Input: part model. Units: mm. Frame: model coordinates. A direction names the side the tool comes from. Round coordinates to 2 decimals unless told otherwise and drop trailing zeros. Loops run counter-clockwise (first coordinate to the right, second up) from the corner with the lowest first, then second, coordinate; pieces in that order, holes last. Notation, with made-up numbers: (-32, 20) -> (-15, 20) arc R16 ccw to (-15, 50) -> close; hole circle Ø6 at (25.25, 24). An arc over 180 degrees is marked (long way). Answer in a Markdown table with one row per item. Add a question column.
Q1. Reachability of faces 1 (the face through (10, 53.34, 10)), 2 (the face through (-22.33, 59.6, 21.93)), 3 (the face through (0.251, 9.396, 29.936)) from +Z, -Z, +X, -X, +Y, -Y: full face, straight path, thin tool, end or side. Return the list, or none.
Q2. Pin query (flat end, axial travel): pin 1 (4 mm diameter, centred on y = 5, z = -5.5, fed in from +X); pin 2 (6 mm diameter, centred on x = -3.5, y = 28, fed in from +Z); pin 3 (4 mm diameter, centred on x = -5.5, y = 2.5, fed in from +Z); pin 4 (8 mm diameter, centred on x = 0, z = -35.92, fed in from +Y). Return the tip coordinate at first contact, or that it passes through.
Q3. Mould query, pull axis X, two halves, no side actions, for faces 4 (the face through (-0.251, 9.396, -29.936)), 5 (the face through (-48.62, 59.6, -0.23)), 6 (the face through (13.52, 5.01, -18.16)). Classes: pulls with the +X half, pulls with the -X half, needs draft (parallel to the pull), parting line crosses it, or undercut.
Q4. Section C-C, the plane y = 38. Output: boundary loops of the cut face in (x, z) (3 decimals), and give its area (3 significant figures).
Q5. Ray query, L1, parallel to Y at x = -11, z = -9.5; L2, parallel to Z at x = 0, y = 26.5 (3 decimals); L3, parallel to Z at x = 33.5, y = 54.5. Return the intervals inside material, ascending. Write a range as from..to.
Q6. Section A-A, the plane x = 0. Give the number of separate pieces and of enclosed holes in the cut face, and give its area (3 significant figures).
Q7. Section D-D, the plane z = -43. Output: boundary loops of the cut face in (x, y), and give its area (3 significant figures).
```python
from build123d import *

# Parameters (mm, degrees)
SKETCH1_R           = 4.445
BOSS_EXTRUDE1_DEPTH = 10.16
FILLET1_R           = 2.54
SKETCH2_R           = 13.97
BOSS_EXTRUDE2_DEPTH = 43.18
SKETCH10_R          = 4.445
BOSS_EXTRUDE3_DEPTH = 12.7
SKETCH11_R          = 9.525
CUT_EXTRUDE1_DEPTH  = 67.04


with BuildPart() as part:
    # Sketch1 → Boss-Extrude1 (new body)
    with BuildSketch(Plane(origin=(0, 0, 0), x_dir=(1, 0, 0), z_dir=(0, 1, 0))):
        with BuildLine():
            Line((-17.960467, -30.660467), (17.960467, -30.660467))
            ThreePointArc((17.960467, -30.660467), (26.940723121, -26.940723121), (30.660467, -17.960467))
            Line((30.660467, -17.960467), (30.660467, 17.960467))
            ThreePointArc((30.660467, 17.960467), (26.940723121, 26.940723121), (17.960467, 30.660467))
            Line((17.960467, 30.660467), (-17.960467, 30.660467))
            ThreePointArc((-17.960467, 30.660467), (-26.940723121, 26.940723121), (-30.660467, 17.960467))
            Line((-30.660467, 17.960467), (-30.660467, -17.960467))
            ThreePointArc((-30.660467, -17.960467), (-26.940723121, -26.940723121), (-17.960467, -30.660467))
        make_face()
        with Locations((-17.960467, 17.960467)):
            Circle(SKETCH1_R, mode=Mode.SUBTRACT)
        with Locations((17.960467, 17.960467)):
            Circle(SKETCH1_R, mode=Mode.SUBTRACT)
        with Locations((-17.960467, -17.960467)):
            Circle(SKETCH1_R, mode=Mode.SUBTRACT)
        with Locations((17.960467, -17.960467)):
            Circle(SKETCH1_R, mode=Mode.SUBTRACT)
    extrude(amount=BOSS_EXTRUDE1_DEPTH)

    # Fillet1
    fillet1_edges = [part.edges().sort_by_distance(p)[0] for p in [
        (26.940723121, 10.16, 26.940723121),
        (30.660467, 10.16, 0),
        (26.940723121, 10.16, -26.940723121),
        (0, 10.16, -30.660467),
        (-26.940723121, 10.16, -26.940723121),
        (-30.660467, 10.16, 0),
        (-26.940723121, 10.16, 26.940723121),
        (0, 10.16, 30.660467),
    ]]
    fillet(fillet1_edges, radius=FILLET1_R)

    # Sketch2 → Boss-Extrude2 (add)
    with BuildSketch(Plane(origin=(0, 10.16, 0), x_dir=(1, 0, 0), z_dir=(0, 1, 0))):
        Circle(SKETCH2_R)
    extrude(amount=BOSS_EXTRUDE2_DEPTH)

    # Sketch10 → Boss-Extrude3 (add)
    with BuildSketch(Plane(origin=(0, 53.34, 0), x_dir=(1, 0, 0), z_dir=(0, 1, 0))):
        with BuildLine():
            ThreePointArc((-39.208026357, 12.267257994), (-48.621024484, 0), (-39.208026357, -12.267257994))
            ThreePointArc((-39.208026357, -12.267257994), (-22.128263612, -22.128263612), (-12.267257994, -39.208026357))
            ThreePointArc((-12.267257994, -39.208026357), (0, -48.621024484), (12.267257994, -39.208026357))
            ThreePointArc((12.267257994, -39.208026357), (22.128263612, -22.128263612), (39.208026357, -12.267257994))
            ThreePointArc((39.208026357, -12.267257994), (48.621024484, 0), (39.208026357, 12.267257994))
            ThreePointArc((39.208026357, 12.267257994), (22.128263612, 22.128263612), (12.267257994, 39.208026357))
            ThreePointArc((12.267257994, 39.208026357), (0, 48.621024484), (-12.267257994, 39.208026357))
            ThreePointArc((-12.267257994, 39.208026357), (-22.128263612, 22.128263612), (-39.208026357, 12.267257994))
        make_face()
        with Locations((-35.921024484, 0)):
            Circle(SKETCH10_R, mode=Mode.SUBTRACT)
        with Locations((0, 35.921024484)):
            Circle(SKETCH10_R, mode=Mode.SUBTRACT)
        with Locations((35.921024484, 0)):
            Circle(SKETCH10_R, mode=Mode.SUBTRACT)
        with Locations((0, -35.921024484)):
            Circle(SKETCH10_R, mode=Mode.SUBTRACT)
    extrude(amount=BOSS_EXTRUDE3_DEPTH)

    # Sketch11 → Cut-Extrude1 (cut, through all)
    with BuildSketch(Plane(origin=(0, 66.04, 0), x_dir=(1, 0, 0), z_dir=(0, 1, 0))):
        Circle(SKETCH11_R)
    extrude(amount=-CUT_EXTRUDE1_DEPTH, mode=Mode.SUBTRACT)

    # Sketch13 → Cut-Revolve1 (revolve, cut)
    with BuildSketch(Plane.XY):
        Polygon((21.59, 66.04), (19.05, 63.5), (0, 63.5), (0, 66.04), align=None)
    revolve(axis=Axis((0, 63.5, 0), (0, 1, 0)), mode=Mode.SUBTRACT)


solid = part.part
```
Answer block:
| question | item | result |
|---|---|---|
| 1 | face 1 | none |
| 1 | face 2 | +Z, -X, +Y |
| 1 | face 3 | +Z, +X, -X |
| 2 | pin 1 | x = 30.66 |
| 2 | pin 2 | z = 13.96 |
| 2 | pin 3 | z = 30.66 |
| 2 | pin 4 | through |
| 3 | face 4 | needs draft |
| 3 | face 5 | pulls with the -X half |
| 3 | face 6 | undercut |
| 4 | outline | circle Ø27.94 at (0, 0); hole circle Ø19.05 at (0, 0) |
| 4 | area | 328 mm^2 |
| 5 | L1 | 0..10.16, 53.34..63.5 |
| 5 | L2 | -13.97..-9.525, 9.525..13.97 |
| 5 | L3 | -14.3..-3.73, 3.73..14.3 |
| 6 | separate pieces | 4 |
| 6 | enclosed holes | 0 |
| 6 | area | 1,520 mm^2 |
| 7 | outline | (-10.54, 53.34) -> (10.54, 53.34) -> (10.54, 66.04) -> (-10.54, 66.04) -> close |
| 7 | area | 268 mm^2 |
